Input: part model. Units: mm. Frame: model coordinates. A direction names the side the tool comes from. Give positions to 0.01 mm unless a question says otherwise; leave off trailing zeros. Order: outer loops, then holes, each group sorted by start corner. A loop starts at its lowest first (then second) coordinate and runs counter-clockwise, first axis right, second up. Notation, with made-up numbers: M 2,10 L 39,10 A20 ccw 39,15 Z; hole C 4,77 d1. An arc over 180 degrees is marked long. Use a Markdown table: item, result.
from build123d import *

# Parameters (mm, degrees)
F1_DEPTH = 2.54
F2_DEPTH = 27.94
F3_DEPTH = 17.78


with BuildPart() as f1:
    # F0 (on Right) → F1 (new body)
    with BuildSketch(Plane.YZ):
        with BuildLine():
            ThreePointArc((0, -19.05), (13.4703841816, -13.4703841816), (19.05, 0))
            ThreePointArc((19.05, 0), (18.748751681, 3.3744348271), (17.854534341, 6.6421459987))
            Line((17.854534341, 6.6421459987), (1.5875, -2.749630657))
            Line((1.5875, -2.749630657), (1.27, -2.1997045256))
            ThreePointArc((1.27, -2.1997045256), (0.6574003746, -2.4534515988), (0, -2.54))
            Line((0, -2.54), (0, -19.05))
        make_face()
        with BuildLine():
            Line((1.5875, -2.749630657), (17.854534341, 6.6421459987))
            ThreePointArc((17.854534341, 6.6421459987), (17.2365354597, 8.1119877556), (16.4977839421, 9.525))
            Line((16.4977839421, 9.525), (2.1997045256, 1.27))
            ThreePointArc((2.1997045256, 1.27), (2.4534515988, 0.6574003746), (2.54, 0))
            ThreePointArc((2.54, 0), (2.1997045256, -1.27), (1.27, -2.1997045256))
            Line((1.27, -2.1997045256), (1.5875, -2.749630657))
        make_face()
        with BuildLine():
            ThreePointArc((16.4977839421, 9.525), (17.2365354597, 8.1119877556), (17.854534341, 6.6421459987))
            Line((17.854534341, 6.6421459987), (31.0085480301, 14.236619343))
            Line((31.0085480301, 14.236619343), (28.0462327016, 16.1925))
            Line((28.0462327016, 16.1925), (16.4977839421, 9.525))
        make_face()
        with BuildLine():
            Line((0, -32.385), (0, -19.05))
            ThreePointArc((0, -19.05), (-1.5930802583, -18.9832714591), (-3.175, -18.7835533113))
            Line((-3.175, -18.7835533113), (-3.175, -33.9725))
            Line((-3.175, -33.9725), (0, -32.385))
        make_face()
        with BuildLine():
            ThreePointArc((-3.175, -18.7835533113), (-1.5930802583, -18.9832714591), (0, -19.05))
            Line((0, -19.05), (0, -2.54))
            ThreePointArc((0, -2.54), (-1.7960512242, -1.7960512242), (-2.54, 0))
            Line((-2.54, 0), (-3.175, 0))
            Line((-3.175, 0), (-3.175, -18.7835533113))
        make_face()
        with BuildLine():
            Line((2.1997045256, 1.27), (16.4977839421, 9.525))
            ThreePointArc((16.4977839421, 9.525), (1.5930802583, 18.9832714591), (-14.679534341, 12.1414073127))
            Line((-14.679534341, 12.1414073127), (1.5875, 2.749630657))
            Line((1.5875, 2.749630657), (1.27, 2.1997045256))
            ThreePointArc((1.27, 2.1997045256), (1.7960512242, 1.7960512242), (2.1997045256, 1.27))
        make_face()
        Polygon((28.0462327016, 16.1925), (31.0085480301, 14.236619343), (32.3833633586, 15.030369343), (30.7958633586, 17.78), align=None)
        Polygon((32.3833633586, 15.030369343), (31.0085480301, 14.236619343), (33.9708633586, 12.280738686), align=None)
        with BuildLine():
            ThreePointArc((-16.4977839421, 9.525), (-17.2365354597, -8.1119877556), (-3.175, -18.7835533113))
            Line((-3.175, -18.7835533113), (-3.175, 0))
            Line((-3.175, 0), (-2.54, 0))
            ThreePointArc((-2.54, 0), (-2.4534515988, 0.6574003746), (-2.1997045256, 1.27))
            Line((-2.1997045256, 1.27), (-16.4977839421, 9.525))
        make_face()
        Polygon((10.5906598886, -24.9693401114), (0, -32.385), (0, -35.56), align=None)
        Polygon((0, -35.56), (0, -32.385), (-3.175, -33.9725), (-3.175, -35.56), align=None)
        with BuildLine():
            Line((1.5875, 2.749630657), (-14.679534341, 12.1414073127))
            ThreePointArc((-14.679534341, 12.1414073127), (-15.6434552014, 10.8712837035), (-16.4977839421, 9.525))
            Line((-16.4977839421, 9.525), (-2.1997045256, 1.27))
            ThreePointArc((-2.1997045256, 1.27), (-0.6574003746, 2.4534515988), (1.27, 2.1997045256))
            Line((1.27, 2.1997045256), (1.5875, 2.749630657))
        make_face()
        with BuildLine():
            ThreePointArc((-16.4977839421, 9.525), (-15.6434552014, 10.8712837035), (-14.679534341, 12.1414073127))
            Line((-14.679534341, 12.1414073127), (-27.8335480301, 19.735880657))
            Line((-27.8335480301, 19.735880657), (-28.0462327016, 16.1925))
            Line((-28.0462327016, 16.1925), (-16.4977839421, 9.525))
        make_face()
        Polygon((16.3287529078, 21.6564505621), (28.0462327016, 16.1925), (30.7958633586, 17.78), align=None)
        Polygon((-3.175, -35.56), (-3.175, -33.9725), (-6.35, -35.56), align=None)
        Polygon((-28.0462327016, 16.1925), (-27.8335480301, 19.735880657), (-29.2083633586, 20.529630657), (-30.7958633586, 17.78), align=None)
        Polygon((-29.2083633586, 20.529630657), (-27.8335480301, 19.735880657), (-27.6208633586, 23.279261314), align=None)
        Polygon((-26.9194127965, 3.3128895493), (-28.0462327016, 16.1925), (-30.7958633586, 17.78), align=None)
    extrude(amount=F1_DEPTH)

    # F0 (on Right) → F2 (join)
    with BuildSketch(Plane.YZ):
        with BuildLine():
            Line((-2.1997045256, 1.27), (0, 0))
            Line((0, 0), (1.27, 2.1997045256))
            ThreePointArc((1.27, 2.1997045256), (-0.6574003746, 2.4534515988), (-2.1997045256, 1.27))
        make_face()
        with BuildLine():
            ThreePointArc((-2.1997045256, 1.27), (-2.4534515988, 0.6574003746), (-2.54, 0))
            Line((-2.54, 0), (0, 0))
            Line((0, 0), (-2.1997045256, 1.27))
        make_face()
        with BuildLine():
            ThreePointArc((-2.54, 0), (-1.7960512242, -1.7960512242), (0, -2.54))
            Line((0, -2.54), (0, 0))
            Line((0, 0), (-2.54, 0))
        make_face()
        with BuildLine():
            Line((0, 0), (0, -2.54))
            ThreePointArc((0, -2.54), (0.6574003746, -2.4534515988), (1.27, -2.1997045256))
            Line((1.27, -2.1997045256), (0, 0))
        make_face()
        with BuildLine():
            ThreePointArc((2.54, 0), (2.4534515988, 0.6574003746), (2.1997045256, 1.27))
            Line((2.1997045256, 1.27), (0, 0))
            Line((0, 0), (1.27, -2.1997045256))
            ThreePointArc((1.27, -2.1997045256), (2.1997045256, -1.27), (2.54, 0))
        make_face()
        with BuildLine():
            Line((0, 0), (2.1997045256, 1.27))
            ThreePointArc((2.1997045256, 1.27), (1.7960512242, 1.7960512242), (1.27, 2.1997045256))
            Line((1.27, 2.1997045256), (0, 0))
        make_face()
    extrude(amount=F2_DEPTH)

    # F0 (on Right) → F3 (join)
    with BuildSketch(Plane.YZ):
        with BuildLine():
            ThreePointArc((2.54, 0), (2.4534515988, 0.6574003746), (2.1997045256, 1.27))
            Line((2.1997045256, 1.27), (0, 0))
            Line((0, 0), (1.27, -2.1997045256))
            ThreePointArc((1.27, -2.1997045256), (2.1997045256, -1.27), (2.54, 0))
        make_face()
        with BuildLine():
            Line((0, 0), (0, -2.54))
            ThreePointArc((0, -2.54), (0.6574003746, -2.4534515988), (1.27, -2.1997045256))
            Line((1.27, -2.1997045256), (0, 0))
        make_face()
        with BuildLine():
            ThreePointArc((-2.54, 0), (-1.7960512242, -1.7960512242), (0, -2.54))
            Line((0, -2.54), (0, 0))
            Line((0, 0), (-2.54, 0))
        make_face()
        with BuildLine():
            ThreePointArc((-2.1997045256, 1.27), (-2.4534515988, 0.6574003746), (-2.54, 0))
            Line((-2.54, 0), (0, 0))
            Line((0, 0), (-2.1997045256, 1.27))
        make_face()
        with BuildLine():
            Line((-2.1997045256, 1.27), (0, 0))
            Line((0, 0), (1.27, 2.1997045256))
            ThreePointArc((1.27, 2.1997045256), (-0.6574003746, 2.4534515988), (-2.1997045256, 1.27))
        make_face()
        with BuildLine():
            Line((0, 0), (2.1997045256, 1.27))
            ThreePointArc((2.1997045256, 1.27), (1.7960512242, 1.7960512242), (1.27, 2.1997045256))
            Line((1.27, 2.1997045256), (0, 0))
        make_face()
    extrude(amount=-F3_DEPTH)


solid = f1.part
1) Cut plane D-D on y = 13.5. Return loops of the section in (x, z), and give its area (3 significant figures).
Response values:
| item | result |
|---|---|
| outline | M 0,-13.44 L 2.54,-13.44 L 2.54,13.44 L 0,13.44 Z |
| area | 68.3 mm² |
2) Mould query, pull axis Z, two halves, no side actions, for faces 4 (the face through (1.3, 32.4, 15)), 5 (the face through (2.54, 1, 3)), 6 (the face through (1.25, 22.11, 18.96)), 7 (the face through (1.25, 5.22, -30.34)). Classes: released by +Z, released by -Z, zero draft, split by the parting line, or undercut.
Response values:
| item | result |
|---|---|
| face 4 | released by +Z |
| face 5 | zero draft |
| face 6 | undercut |
| face 7 | released by -Z |
3) Material intervals for line 1 (X direction, y = -14.5, z = 1.5); line 2 (Z direction, x = 0.5, y = 31); line 3 (Z direction, x = -9, y = -1), sorted ascending. Write a range as from..to.
Response values:
| item | result |
|---|---|
| line 1 | x = 0..2.54 |
| line 2 | z = 14.23..17.43 |
| line 3 | z = -2.33..2.33 |
4) First-contact query: pin 1 Ø10 at (y, z) = (-7, -22) entering from +X; pin 2 Ø0.8 at (x, z) = (2, -23.5) entering from -Y (3 decimals); pin 3 Ø0.8 at (x, z) = (1, -22.5) entering from +Y. Flat tips, straight axial feed; report the tip coordinate or a pass-through.
Response values:
| item | result |
|---|---|
| pin 1 | stops at x = 2.54 |
| pin 2 | stops at y = -3.175 |
| pin 3 | stops at y = 0 |
5) Cut plane C-C on z = 8.5. Return loops of the section in (x, y).
Response values:
| item | result |
|---|---|
| outline | M 0,-28.31 L 2.54,-28.31 L 2.54,-27.37 L 0,-27.37 Z; M 0,-17.05 L 2.54,-17.05 L 2.54,21.07 L 0,21.07 Z |
6) Cut plane B-B on y = 4. Return loops of the section in (x, z), and give its area (3 significant figures).
Response values:
| item | result |
|---|---|
| outline | M 0,-31.56 L 2.54,-31.56 L 2.54,-29.58 L 0,-29.58 Z; M 0,-18.63 L 2.54,-18.63 L 2.54,18.63 L 0,18.63 Z |
| area | 99.6 mm² |
7) Cut plane A-A on x = 5. Return loops of the section in (y, z).
Response values:
| item | result |
|---|---|
| outline | C 0,0 d5.08 |
8) Reachability of faces 1 (the face through (1.25, 32.47, 13.27)), 2 (the face through (1.252, -29.186, 20.568)), 3 (the face through (1.252, 22.353, 12.905)) from +Z, -Z, +X, -X, +Y, -Y: full face, straight path, thin tool, end or side. Return the list, or none.
Response values:
| item | result |
|---|---|
| face 1 | -Z, +X, -X |
| face 2 | +Z, +X, -X, -Y |
| face 3 | +X, -X |
